from build123d import *

# Parameters (mm, degrees)
SKETCH_1_R          = 49
EXTRUDE_1_DEPTH     = 30
FILLET_1_R          = 3
SKETCH_2_R          = 21
CUT_EXTRUDE_1_DEPTH = 6
SKETCH_3_R          = 2.5
CUT_EXTRUDE_2_DEPTH = 6


with BuildPart() as part:
    # 草图1 → 凸台-拉伸1 (new body)
    with BuildSketch(Plane(origin=(0, 0, 0), x_dir=(0, 0, -1), z_dir=(1, 0, 0))):
        Circle(SKETCH_1_R)
    extrude(amount=EXTRUDE_1_DEPTH)

    # 圆角1
    fillet_1_edges = [part.edges().sort_by_distance(p)[0] for p in [
        (0, 0, 49),
        (30, 0, 49),
    ]]
    fillet(fillet_1_edges, radius=FILLET_1_R)

    # 草图2 → 切除-拉伸1 (cut)
    with BuildSketch(Plane(origin=(30, 0, 0), x_dir=(0, 0, -1), z_dir=(1, 0, 0))):
        Circle(SKETCH_2_R)
    extrude(amount=-CUT_EXTRUDE_1_DEPTH, mode=Mode.SUBTRACT)

    # 草图3 → 切除-拉伸2 (cut)
    with BuildSketch(Plane(origin=(24, 0, 0), x_dir=(0, 0, -1), z_dir=(1, 0, 0))):
        Circle(SKETCH_3_R)
    extrude(amount=-CUT_EXTRUDE_2_DEPTH, mode=Mode.SUBTRACT)


solid = part.part
The listing builds one solid part. Answer for the finished solid, in the listing's coordinates (mm). A direction names the side the tool comes from. Give positions to 0.01 mm unless a question says otherwise; leave off trailing zeros. Order: outer loops, then holes, each group sorted by start corner. A loop starts at its lowest first (then second) coordinate and runs counter-clockwise, first axis right, second up. Notation, with made-up numbers: (0, -10.75) -> (59, -10.75) arc R37 cw to (59, 27.25) -> close; hole circle Ø11 at (62.25, 4.5). An arc over 180 degrees is marked (long way). Put each result on its own line as item: value.
Item 1: A cutting plane is placed at C-C on x = 20. Give the vertices of the cut face in (y, z), plus the area to 3 significant figures.
Established:
outline: circle Ø98 at (0, 0); hole circle Ø5 at (0, 0)
area: 7,520 mm^2
Item 2: For faces 1 (the face through (0, 1, 1)), 2 (the face through (27.04, 6.31, -20.03)), determine the directions among +Z, -Z, +X, -X, +Y, -Y from which every point of the face is accessible in a straight line to the end or side of a thin tool.
Established:
face 1: +Z, -Z, -X, +Y, -Y
face 2: +X
Item 3: For a pull along Y with two mould halves and no side action, classify faces 3 (the face through (24, 0, -4)), 4 (the face through (30, -10, -20)), 5 (the face through (14.83, 41.32, -26.34)) as released by +Y, released by -Y, zero draft, split by the parting line, or undercut.
Established:
face 3: undercut
face 4: zero draft
face 5: split by the parting line
Item 4: Straight lines are drawn through the part: line 1 (Y direction, x = 26.45, z = 0); line 2 (X direction, y = -17, z = 8); line 3 (Z direction, x = 13.75, y = -0.5). For each, find the intervals that lie inside material, in ascending order.
Established:
line 1: y = -49 to -21, 21 to 49
line 2: x = 0 to 24
line 3: z = -49 to 49
Item 5: A cutting plane is placed at A-A on z = 0. Give the vertices of the cut face in (x, y).
Established:
outline: (0, -46) arc R3 ccw to (3, -49) -> (27, -49) arc R3 ccw to (30, -46) -> (30, -21) -> (24, -21) -> (24, -2.5) -> (18, -2.5) -> (18, 2.5) -> (24, 2.5) -> (24, 21) -> (30, 21) -> (30, 46) arc R3 ccw to (27, 49) -> (3, 49) arc R3 ccw to (0, 46) -> close
Item 6: Given P1, Ø4, axis at x = 19.5, y = -36, coming from the -Z side; P2, Ø6, axis at y = 0, z = 0, coming from the +X side; P3, Ø1.5, axis at x = 11, z = -0.5, coming from the -Y side, each flat-ended and moving along its own axis, determine where each tip first touches the part or whether it passes through.
Established:
P1: stops at z = -35.28
P2: stops at x = 24
P3: stops at y = -49
